Check sheet for the modelled part. Datum: model origin and axes. Units: mm. Face numbers are marked on the shaded views. Give positions to 0.01 mm unless a question says otherwise; leave off trailing zeros. Order: outer loops, then holes, each group sorted by start corner. A loop starts at its lowest first (then second) coordinate and runs counter-clockwise, first axis right, second up. Notation, with made-up numbers: (44.25, 48.5) -> (93.25, 48.5) arc R18 ccw to (93.25, 68.5) -> close; hole circle Ø4 at (-5.75, 43). An arc over 180 degrees is marked (long way). One line per question, with ' | ' between items. Start each with the question number.
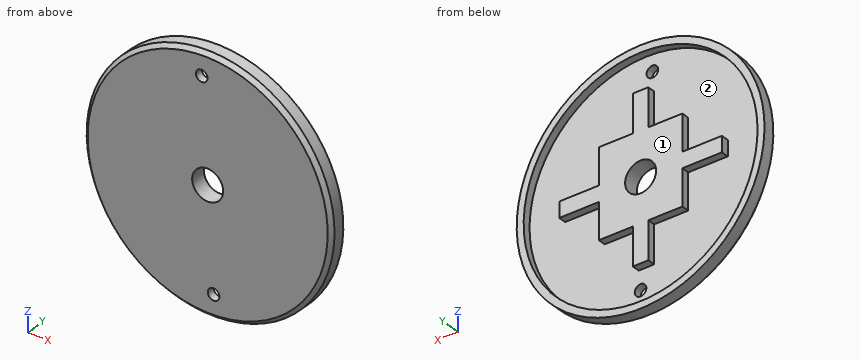
from build123d import *

# Parameters (mm, degrees)
SKETCH1_R           = 32
BOSS_EXTRUDE1_DEPTH = 4
SKETCH2_R           = 30.2
CUT_EXTRUDE1_DEPTH  = 2
CHAMFER1_SIZE       = 1
SKETCH3_R           = 1.5
CUT_EXTRUDE2_DEPTH  = 15
SKETCH5_W           = 4
SKETCH5_H           = 42
SKETCH5_W_2         = 42
SKETCH5_H_2         = 4
BOSS_EXTRUDE2_DEPTH = 2
SKETCH6_R           = 4
CUT_EXTRUDE3_DEPTH  = 10
SKETCH7_W           = 15
SKETCH7_H           = 20
CUT_EXTRUDE4_DEPTH  = 10
BOSS_EXTRUDE3_START = 2
SKETCH8_W           = 21.56425071
SKETCH8_H           = 22.582305464
SKETCH8_R           = 4
BOSS_EXTRUDE3_DEPTH = 2


with BuildPart() as part:
    # Sketch1 → Boss-Extrude1 (new body)
    with BuildSketch(Plane(origin=(0, 0, 0), x_dir=(1, 0, 0), z_dir=(0, 1, 0))):
        with Locations(Location((0, 0, 0), (0, 0, 270))):
            Circle(SKETCH1_R)
    extrude(amount=BOSS_EXTRUDE1_DEPTH)

    # Sketch2 → Cut-Extrude1 (cut)
    with BuildSketch(Plane(origin=(0, 4, 0), x_dir=(1, 0, 0), z_dir=(0, 1, 0))):
        with Locations(Location((0, 0, 0), (0, 0, 270))):
            Circle(SKETCH2_R)
    extrude(amount=-CUT_EXTRUDE1_DEPTH, mode=Mode.SUBTRACT)

    # Chamfer1
    chamfer1_edges = [part.edges().sort_by_distance(p)[0] for p in [
        (0, 0, -32),
    ]]
    chamfer(chamfer1_edges, length=CHAMFER1_SIZE)

    # Sketch3 → Cut-Extrude2 (cut)
    with BuildSketch(Plane.XZ):
        with Locations(Location((-1.532005462, 25.954825356, 0), (0, 0, 270))):
            Circle(SKETCH3_R)
        with Locations(Location((1.532016667, -25.954824695, 0), (0, 0, 270))):
            Circle(SKETCH3_R)
    extrude(amount=-CUT_EXTRUDE2_DEPTH, mode=Mode.SUBTRACT)

    # Sketch5 → Boss-Extrude2 (add)
    with BuildSketch(Plane(origin=(0, 2, 0), x_dir=(1, 0, 0), z_dir=(0, 1, 0))):
        Rectangle(SKETCH5_W, SKETCH5_H)
        Rectangle(SKETCH5_W_2, SKETCH5_H_2)
    extrude(amount=BOSS_EXTRUDE2_DEPTH)

    # Sketch6 → Cut-Extrude3 (cut)
    with BuildSketch(Plane(origin=(0, 4, 0), x_dir=(1, 0, 0), z_dir=(0, 1, 0))):
        with Locations(Location((0, 0, 0), (0, 0, 270))):
            Circle(SKETCH6_R)
    extrude(amount=-CUT_EXTRUDE3_DEPTH, mode=Mode.SUBTRACT)

    # Sketch7 → Cut-Extrude4 (cut)
    with BuildSketch(Plane(origin=(0, 2, 0), x_dir=(1, 0, 0), z_dir=(0, 1, 0))):
        Rectangle(SKETCH7_W, SKETCH7_H)
    extrude(amount=CUT_EXTRUDE4_DEPTH, mode=Mode.SUBTRACT)

    # Sketch8 → Boss-Extrude3 (add)
    with BuildSketch(Plane(origin=(0, 2, 0), x_dir=(1, 0, 0), z_dir=(0, 1, 0)).offset(BOSS_EXTRUDE3_START)):
        Rectangle(SKETCH8_W, SKETCH8_H)
        with Locations(Location((0, 0, 0), (0, 0, 270))):
            Circle(SKETCH8_R, mode=Mode.SUBTRACT)
    extrude(amount=-BOSS_EXTRUDE3_DEPTH)


solid = part.part
1. Scan lines: probe 1 along X at (y, z) = (1.1, 0); probe 2 along X at (y, z) = (3.1, 0); probe 3 along Z at (x, y) = (1, 0.4). Record each from-to range of solid material in increasing order.
2. Cross-section at A-A on y = 3.35. Record the boundary of the cut face in (x, z).
3. Cross-section at B-B on z = 0. Record the boundary of the cut face in (x, y).
4. Mould release check, pull along Z, two halves, no side actions. Record for the marked faces 1 and 2: +Z half, -Z half, draft (parallel to the pull), parting line (faces both ways), or undercut.
5. Go/stop test with flat-tipped pins: pin 1 (0.6 mm diameter, centred on y = 3.5, z = 17.5, fed in from +X); pin 2 (1.5 mm diameter, centred on y = 1.5, z = -22.5, fed in from +X); pin 3 (0.6 mm diameter, centred on y = 3, z = 0, fed in from +X). Record where each tip stops, or that it passes through.
Response values:
1) probe 1: x = -32 to -4, 4 to 32 | probe 2: x = -32 to -30.2, -21 to -4, 4 to 21, 30.2 to 32 | probe 3: z = -31.38 to -27.36, -24.55 to -3.87, 3.87 to 31.38
2) outline: circle Ø64 at (0, 0); (-21, -2) -> (-10.78, -2) -> (-10.78, -11.29) -> (-2, -11.29) -> (-2, -21) -> (2, -21) -> (2, -11.29) -> (10.78, -11.29) -> (10.78, -2) -> (21, -2) -> (21, 2) -> (10.78, 2) -> (10.78, 11.29) -> (2, 11.29) -> (2, 21) -> (-2, 21) -> (-2, 11.29) -> (-10.78, 11.29) -> (-10.78, 2) -> (-21, 2) -> close; hole circle Ø60.4 at (0, 0); hole circle Ø8 at (0, 0)
3) outline: (-32, 1) -> (-31, 0) -> (-4, 0) -> (-4, 4) -> (-21, 4) -> (-21, 2) -> (-30.2, 2) -> (-30.2, 4) -> (-32, 4) -> close; (4, 0) -> (31, 0) -> (32, 1) -> (32, 4) -> (30.2, 4) -> (30.2, 2) -> (21, 2) -> (21, 4) -> (4, 4) -> close
4) face 1: draft | face 2: undercut
5) pin 1: stops at x = 26.98 | pin 2: stops at x = 23.47 | pin 3: stops at x = 32
